The model under review builds one solid part; all positions refer to its coordinate system, in mm. A direction names the side the tool comes from. Round coordinates to 2 decimals unless told otherwise and drop trailing zeros. Order: outer loops, then holes, each group sorted by start corner. A loop starts at its lowest first (then second) coordinate and runs counter-clockwise, first axis right, second up. Notation, with made-up numbers: M 69,24.25 L 94,24.25 A12 ccw 94,43.25 Z; hole C -38.5,32.5 d2. An arc over 180 degrees is marked long. Answer as a JSON object with one key per item and string values. Group by question number.
1. Add section A-A on y = -5. State the section outline as (x, z) points, and give its area (3 significant figures).
2. Mouldability with a two-part tool opening along Y and no side actions: class faces 3 (the face through (-1, 25, 12)), 4 (the face through (-1, 20, 15)), 5 (the face through (17.968, -5.843, 2.465)) as released by +Y, released by -Y, zero draft, split by the parting line, or undercut.
3. Add section C-C on z = 11.5. State the section outline as (x, y) points, and give its area (3 significant figures).
4. To check wall thickness, follow probe 1 along Y at (x, z) = (20, 4); probe 2 along Z at (x, y) = (15, -13); probe 3 along Y at (x, z) = (-6, 21). State the ranges of each line that lie inside material, in increasing order. Write a range as [from, to].
5. Clearance check with a flat-ended pin moving along its axis: P1, Ø2, axis at x = -26.5, y = -15, coming from the +Z side. State where the tip first meets the part, or that it passes through.
6. Machinability: for faces 1 (the face through (-1, -2, 5)), 2 (the face through (-1, 0, 0)), which of the approach directions +Z, -Z, +X, -X, +Y, -Y give a long, thin tool a straight path to every point of the face, cutting with its end or side? Answer none if there is none.
7. Add section B-B on x = 20. State the section outline as (y, z) points, and give its area (3 significant figures).
```python
from build123d import *

# Parameters (mm, degrees)
F0_W     = 80
F0_H     = 50
F1_DEPTH = 5
F2_W     = 80
F2_H     = 5
F3_DEPTH = 20
F5_D     = 4.4


with BuildPart() as f1:
    # F0 (on Top) → F1 (new body)
    with BuildSketch(Plane.XY):
        Rectangle(F0_W, F0_H)
    extrude(amount=F1_DEPTH)

    # F2 (on face) → F3 (join)
    with BuildSketch(Plane.XY.offset(5)):
        with Locations((0, 22.5)):
            Rectangle(F2_W, F2_H)
    extrude(amount=F3_DEPTH)

    # F5 (through all)
    with Locations(Plane.XY.offset(5)):
        with Locations((-20, -5), (20, -5)):
            Hole(F5_D / 2)


solid = f1.part
```
Recorded:
{
 "1": {"outline": "M -40,0 L -22.2,0 L -22.2,5 L -40,5 Z; M -17.8,0 L 17.8,0 L 17.8,5 L -17.8,5 Z; M 22.2,0 L 40,0 L 40,5 L 22.2,5 Z", "area": "356 mm²"},
 "2": {"face 3": "released by +Y", "face 4": "released by -Y", "face 5": "undercut"},
 "3": {"outline": "M -40,20 L 40,20 L 40,25 L -40,25 Z", "area": "400 mm²"},
 "4": {"probe 1": "y = [-25, -7.2], [-2.8, 25]", "probe 2": "z = [0, 5]", "probe 3": "y = [20, 25]"},
 "5": {"P1": "stops at z = 5"},
 "6": {"face 1": "+Z, +X, -X, -Y", "face 2": "-Z, +X, -X, +Y, -Y"},
 "7": {"outline": "M -25,0 L -7.2,0 L -7.2,5 L -25,5 Z; M -2.8,0 L 25,0 L 25,25 L 20,25 L 20,5 L -2.8,5 Z", "area": "328 mm²"}
}
